Input: part model. Units: mm. Frame: model coordinates. Face numbers are marked on the shaded views. A direction names the side the tool comes from. Give positions to 0.01 mm unless a question says otherwise; leave off trailing zeros. Loops run counter-clockwise (first coordinate to the right, second up) from the corner with the lowest first, then second, coordinate; pieces in that order, holes last. Notation, with made-up numbers: (50.5, 28.5) -> (65.5, 28.5) arc R15 ccw to (65.5, 54.5) -> close; hole circle Ø5 at (36.25, -6). An arc over 180 degrees is marked (long way). Answer as a JSON object with one key per item and string values. Group by question number.
```python
from build123d import *

# Parameters (mm, degrees)
BOSS_EXTRUDE1_DEPTH = 94.9452
SKETCH2_R           = 18.923
CUT_EXTRUDE1_DEPTH  = 56.9976
BOSS_EXTRUDE2_START = -2.9972
BOSS_EXTRUDE2_DEPTH = 2.9972
HOLE1_D             = 7.9375


with BuildPart() as part:
    # Sketch1 → Boss-Extrude1 (new body)
    with BuildSketch(Plane.XY):
        with BuildLine():
            Line((21.960352912, 16.51), (41.275, 16.51))
            Line((41.275, 16.51), (41.275, 22.86))
            Line((41.275, 22.86), (15.875, 22.86))
            ThreePointArc((15.875, 22.86), (0, 6.985), (-15.875, 22.86))
            Line((-15.875, 22.86), (-41.275, 22.86))
            Line((-41.275, 22.86), (-41.275, 16.51))
            Line((-41.275, 16.51), (-21.960352912, 16.51))
            ThreePointArc((-21.960352912, 16.51), (0, 0), (21.960352912, 16.51))
        make_face()
    extrude(amount=BOSS_EXTRUDE1_DEPTH)

    # Sketch2 → Cut-Extrude1 (cut)
    with BuildSketch(Plane(origin=(0, 0, 0), x_dir=(-1, 0, 0), z_dir=(0, 0, -1))):
        with Locations((0, 22.86)):
            Circle(SKETCH2_R)
    extrude(amount=-CUT_EXTRUDE1_DEPTH, mode=Mode.SUBTRACT)

    # Sketch3 → Boss-Extrude2 (add)
    with BuildSketch(Plane.XY.offset(94.9452).offset(BOSS_EXTRUDE2_START)):
        with BuildLine():
            Line((-15.875, 22.86), (-9.0043, 22.86))
            Line((-9.0043, 22.86), (-9.0043, 18.521727588))
            ThreePointArc((-9.0043, 18.521727588), (0, 12.8651), (9.0043, 18.521727588))
            Line((9.0043, 18.521727588), (9.0043, 22.86))
            Line((9.0043, 22.86), (15.875, 22.86))
            ThreePointArc((15.875, 22.86), (0, 6.985), (-15.875, 22.86))
        make_face()
    extrude(amount=BOSS_EXTRUDE2_DEPTH)

    # Hole1 (through all)
    with Locations(Plane(origin=(0, 16.51, 0), x_dir=(-1, 0, 0), z_dir=(0, -1, 0))):
        with Locations((30.099, -32.004), (30.099, -82.2452)):
            hole1 = Hole(HOLE1_D / 2)

    # Mirror1: Hole1 across plane
    add(hole1.mirror(Plane(origin=(0, 0, 0), x_dir=(0, 0, 1), z_dir=(1, 0, 0))), mode=Mode.SUBTRACT)


solid = part.part
```
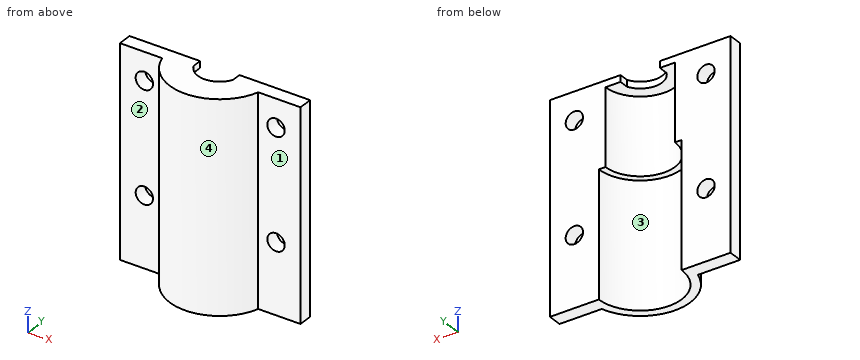
Q1. Pin query (flat end, axial travel): pin 1 Ø5 at (x, y) = (7.5, 16) entering from -Z; pin 2 Ø4 at (y, z) = (12.5, 33.5) entering from +X; pin 3 Ø6 at (x, z) = (-24, 42) entering from -Y; pin 4 Ø5 at (x, z) = (-30.1, 82.25) entering from -Y. Return the tip coordinate at first contact, or that it passes through.
Q2. Section D-D on z = 80. Return the cut outline in (x, y) (3 decimals), then the cut area to 3 significant figures.
Q3. Ray query, probe 1 along Y at (x, z) = (27, 4.5); probe 2 along X at (y, z) = (13.25, 21); probe 3 along X at (y, z) = (13.5, 8.5). Return the intervals inside material, ascending.
Q4. Section A-A on x = -31.5. Return the cut outline in (y, z).
Q5. Section C-C on y = 14.75. Return the cut outline in (x, z), then the cut area to 3 significant figures.
Q6. Set-up query: the marked faces 1, 2, 3 and 4. Return all of +Z, -Z, +X, -X, +Y, -Y with unobstructed straight access to the full face (end or side cutting, diameter ignored); none if empty.
Q7. Section B-B on z = 66.5. Return the cut outline in (x, y) (3 decimals).
Numbers:
{
 "1": {"pin 1": "stops at z = 91.95", "pin 2": "stops at x = 21.28", "pin 3": "stops at y = 13.83", "pin 4": "passes through"},
 "2": {"outline": "(-41.275, 16.51) -> (-33.372, 16.51) -> (-33.372, 22.86) -> (-41.275, 22.86) -> close; (-26.826, 16.51) -> (-21.96, 16.51) arc R22.86 ccw to (21.96, 16.51) -> (26.826, 16.51) -> (26.826, 22.86) -> (15.875, 22.86) arc R15.875 cw to (-15.875, 22.86) -> (-26.826, 22.86) -> close; (33.372, 16.51) -> (41.275, 16.51) -> (41.275, 22.86) -> (33.372, 22.86) -> close", "area": "580 mm²"},
 "3": {"probe 1": "y = 16.51 to 22.86", "probe 2": "x = -20.74 to -16.3, 16.3 to 20.74", "probe 3": "x = -20.86 to -16.45, 16.45 to 20.86"},
 "4": {"outline": "(16.51, 0) -> (22.86, 0) -> (22.86, 28.29) -> (16.51, 28.29) -> close; (16.51, 35.72) -> (22.86, 35.72) -> (22.86, 78.53) -> (16.51, 78.53) -> close; (16.51, 85.96) -> (22.86, 85.96) -> (22.86, 94.95) -> (16.51, 94.95) -> close"},
 "5": {"outline": "(-21.37, 0) -> (-17.1, 0) -> (-17.1, 57) -> (-13.65, 57) -> (-13.65, 91.95) -> (-5.84, 91.95) -> (-5.84, 94.95) -> (-21.37, 94.95) -> close; (5.84, 91.95) -> (13.65, 91.95) -> (13.65, 57) -> (17.1, 57) -> (17.1, 0) -> (21.37, 0) -> (21.37, 94.95) -> (5.84, 94.95) -> close", "area": "1,120 mm²"},
 "6": {"face 1": "+Z, -Z, +X, -Y", "face 2": "+Z, -Z, -X, -Y", "face 3": "-Z, +Y", "face 4": "+Z, -Z, -Y"},
 "7": {"outline": "(-41.275, 16.51) -> (-21.96, 16.51) arc R22.86 ccw to (21.96, 16.51) -> (41.275, 16.51) -> (41.275, 22.86) -> (15.875, 22.86) arc R15.875 cw to (-15.875, 22.86) -> (-41.275, 22.86) -> close"}
}
